```python
from build123d import *

# Parameters (mm, degrees)
SKETCH1_W           = 128.5
SKETCH1_H           = 125
BOSS_EXTRUDE1_DEPTH = 2.4
BOSS_EXTRUDE2_DEPTH = 125
CUT_EXTRUDE2_DEPTH  = 94.975369496
SKETCH6_R           = 1.7
CUT_EXTRUDE3_DEPTH  = 94.975369496


with BuildPart() as part:
    # Sketch1 → Boss-Extrude1 (new body)
    with BuildSketch(Plane(origin=(0, 0, 0), x_dir=(1, 0, 0), z_dir=(0, 1, 0))):
        Rectangle(SKETCH1_W, SKETCH1_H)
    extrude(amount=BOSS_EXTRUDE1_DEPTH)

    # Sketch3 → Boss-Extrude2 (add)
    with BuildSketch(Plane.XY.offset(62.5)):
        Polygon((-64.25, 2.4), (-66.05, 2.4), (-66.15, 2.4), (-66.15, 4.61), (-68.008287326, 4.61), (-70.138149903, 2.458869363), (-70.138149903, 0), (-64.25, 0), align=None)
    extrude(amount=-BOSS_EXTRUDE2_DEPTH)

    # Sketch5 → Cut-Extrude2 (cut, through all)
    with BuildSketch(Plane(origin=(0, 2.4, 0), x_dir=(1, 0, 0), z_dir=(0, 1, 0))):
        with BuildLine():
            Line((-51.25, 47.5), (-51.25, 62.5))
            Line((-51.25, 62.5), (-61.25, 62.5))
            Line((-61.25, 62.5), (-61.25, 47.5))
            ThreePointArc((-61.25, 47.5), (-56.25, 42.5), (-51.25, 47.5))
        make_face()
        with BuildLine():
            Line((-61.25, 62.5), (-51.25, 62.5))
            ThreePointArc((-51.25, 62.5), (-56.25, 67.5), (-61.25, 62.5))
        make_face()
    extrude(amount=-CUT_EXTRUDE2_DEPTH, mode=Mode.SUBTRACT)

    # Sketch6 → Cut-Extrude3 (cut, through all)
    with BuildSketch(Plane(origin=(0, 2.4, 0), x_dir=(1, 0, 0), z_dir=(0, 1, 0))):
        with Locations(Location((-60.25, -59, 0), (0, 0, 270))):
            Circle(SKETCH6_R)
    extrude(amount=-CUT_EXTRUDE3_DEPTH, mode=Mode.SUBTRACT)


solid = part.part
```
Geometry: final body of the model. Coordinates: model frame, mm. A direction names the side the tool comes from. Give positions to 0.01 mm unless a question says otherwise; leave off trailing zeros. Order: outer loops, then holes, each group sorted by start corner. A loop starts at its lowest first (then second) coordinate and runs counter-clockwise, first axis right, second up. Notation, with made-up numbers: M 61.25,47.25 L 113.25,47.25 A17 ccw 113.25,68.25 Z; hole C 78.5,40.25 d1. An arc over 180 degrees is marked long. Answer as CSV lines item,"result". Start each with the question number.
1) First-contact query: P1, Ø0.7, axis at y = 3, z = -6.5, coming from the +X side; P2, Ø3, axis at x = 2.5, z = 23.5, coming from the +Y side; P3, Ø2, axis at x = 21.5, y = 4, coming from the -Z side. Flat tips, straight axial feed; report the tip coordinate or a pass-through.
2) Cut plane C-C (x = 26). Output: boundary loops of the cut face in (y, z), then the cut area to 3 significant figures.
3) Cut plane A-A (z = 59). Output: boundary loops of the cut face in (x, y), then the cut area to 3 significant figures.
4) Set-up query: faces 4 (the flat face through (0, 2.4, 1)), 5 (the flat face through (-4, 0, 1)). Return all of +Z, -Z, +X, -X, +Y, -Y with unobstructed straight access to the full face (end or side cutting, diameter ignored); none if empty.
5) Cut plane D-D (x = -57). Output: boundary loops of the cut face in (y, z).
6) Line query: line 1 (X direction, y = 1.35, z = 59); line 2 (Y direction, x = -48, z = 3.5); line 3 (X direction, y = 2.85, z = -13). Output: solid intervals per line, ascending. Write a range as from..to.
7) Mould query, pull axis Z, two halves, no side actions, for faces 1 (the flat face through (-4, 1, 62.5)), 2 (the cylindrical face through (-56.36, 1.22, -42.5)), 3 (the cylindrical face through (-60.2, 1.2, 57.3)). Classes: +Z half, -Z half, draft (parallel to the pull), parting line (faces both ways), or undercut.
8) Cut plane B-B (z = -51.5). Output: boundary loops of the cut face in (x, y).
Findings below:
1,P1,"stops at x = -66.15"
1,P2,"stops at y = 2.4"
1,P3,"passes through"
2,outline,"M 0,-62.5 L 2.4,-62.5 L 2.4,62.5 L 0,62.5 Z"
2,area,"300 mm²"
3,outline,"M -70.14,0 L -61.95,0 L -61.95,2.4 L -66.15,2.4 L -66.15,4.61 L -68.01,4.61 L -70.14,2.46 Z; M -58.55,0 L 64.25,0 L 64.25,2.4 L -58.55,2.4 Z"
3,area,"321 mm²"
4,face 4,"+Z, -Z, +X, +Y"
4,face 5,"+Z, -Z, +X, -X, -Y"
5,outline,"M 0,-42.56 L 2.4,-42.56 L 2.4,62.5 L 0,62.5 Z"
6,line 1,"x = -70.14..-61.95, -58.55..64.25"
6,line 2,"y = 0..2.4"
6,line 3,"x = -69.75..-66.15"
7,face 1,"+Z half"
7,face 2,"-Z half"
7,face 3,"undercut"
8,outline,"M -70.14,0 L -61.25,0 L -61.25,2.4 L -66.15,2.4 L -66.15,4.61 L -68.01,4.61 L -70.14,2.46 Z; M -51.25,0 L 64.25,0 L 64.25,2.4 L -51.25,2.4 Z"
